```python
from build123d import *

# Parameters (mm, degrees)
CUT_EXTRUDE_1_DEPTH      = 168.620106193
SKETCH_3_R               = 9
CUT_EXTRUDE_2_DEPTH      = 163.450761771
PATTERN_CIRCULAR_1_COUNT = 6


with BuildPart() as part:
    # Эскиз1 → Повернуть1 (revolve)
    with BuildSketch(Plane.XY, mode=Mode.PRIVATE) as revolve_1_sk:
        Polygon((-90.5, 0), (-117.5, 0), (-117.5, -22), (-86.5, -22), (-86.5, -10), (-90.5, -10), align=None)
    revolve(revolve_1_sk.sketch.rotate(Axis((0, 22.934814099, 0), (0, -1, 0)), 270), axis=Axis((0, 22.934814099, 0), (0, -1, 0)))

    # Эскиз2 → Вырез-Вытянуть1 (cut, through all)
    with BuildSketch(Plane(origin=(0, 0, 0), x_dir=(1, 0, 0), z_dir=(0, 1, 0))):
        with BuildLine():
            Line((-110, 41.306779105), (-110, -41.306779105))
            ThreePointArc((-110, -41.306779105), (-117.5, 0), (-110, 41.306779105))
        make_face()
        with BuildLine():
            Line((110, 41.306779105), (110, -41.306779105))
            ThreePointArc((110, -41.306779105), (117.5, 0), (110, 41.306779105))
        make_face()
    extrude(amount=-CUT_EXTRUDE_1_DEPTH, mode=Mode.SUBTRACT)

    # Эскиз3 → Вырез-Вытянуть2 (cut, through all)
    with BuildSketch(Plane(origin=(0, 0, 0), x_dir=(1, 0, 0), z_dir=(0, 1, 0))):
        with Locations(Location((0, 102.5, 0), (0, 0, 270))):
            Circle(SKETCH_3_R)
    cut_extrude_2 = extrude(amount=-CUT_EXTRUDE_2_DEPTH, mode=Mode.SUBTRACT)

    # Круговой массив1: Вырез-Вытянуть2 ×6 about axis
    pattern_circular_1_axis = Axis((0, 0, 0), (0, 1, 0))
    for i in range(1, PATTERN_CIRCULAR_1_COUNT):
        add(cut_extrude_2.rotate(pattern_circular_1_axis, i * 360 / PATTERN_CIRCULAR_1_COUNT), mode=Mode.SUBTRACT)


solid = part.part
```
The listing builds one solid part. Answer for the finished solid, in the listing's coordinates (mm). A direction names the side the tool comes from. Give positions to 0.01 mm unless a question says otherwise; leave off trailing zeros. Write each loop counter-clockwise with the first axis right and the second up, starting at its lowest first coordinate (ties: lowest second). Pieces come first, ordered by that corner, then holes. Notation, with made-up numbers: M 59,11 L 109,11 A34 cw 109,41 Z; hole C -38.5,65.5 d7. An arc over 180 degrees is marked long. Write each question's results on one line, items separated by ' | '.
Q1. Flat-ended cylindrical pins translate along their axes: P1, Ø12, axis at x = 71, y = -19, coming from the -Z side; P2, Ø6, axis at y = -11, z = -78, coming from the -X side; P3, Ø5, axis at x = 36.5, y = -12.5, coming from the +Z side. Find the tip coordinate at first contact, or state that the pin passes through.
Output values:
P1: z = -97.88 | P2: x = -90.45 | P3: z = 112.47
Q2. Consider L1, parallel to X at y = -19.75, z = 57.5; L2, parallel to X at y = -11.25, z = -51.25; L3, parallel to X at y = -14.75, z = 0. Determine where each line is inside the solid, lowest interval first. Write a range as from..to.
Output values:
L1: -102.47..-95.24, -82.29..-64.62, 64.62..82.29, 95.24..102.47 | L2: -105.73..-97.77, -79.77..-69.68, 69.68..79.77, 97.77..105.73 | L3: -110..-86.5, 86.5..110
Q3. Section B-B, the plane x = -32.5 is taken. Write down the section's boundary in (y, z).
Output values:
outline: M -22,-112.92 L 0,-112.92 L 0,-84.46 L -10,-84.46 L -10,-80.16 L -22,-80.16 Z; M -22,80.16 L -10,80.16 L -10,84.46 L 0,84.46 L 0,112.92 L -22,112.92 Z
Q4. Section D-D, the plane y = -17 is taken. Write down the section's boundary in (x, z), then the cut area to 3 significant figures.
Output values:
outline: M -110,-41.31 A117.5 ccw 110,-41.31 L 110,41.31 A117.5 ccw -110,41.31 Z; hole C -88.77,-51.25 d18; hole C -88.77,51.25 d18; hole C 0,0 d173; hole C 0,-102.5 d18; hole C 0,102.5 d18; hole C 88.77,-51.25 d18; hole C 88.77,51.25 d18 | area: 17,500 mm2
Q5. Section A-A, the plane z = 0 is taken. Write down the section's boundary in (x, y), then the cut area to 3 significant figures.
Output values:
outline: M -110,-22 L -86.5,-22 L -86.5,-10 L -90.5,-10 L -90.5,0 L -110,0 Z; M 86.5,-22 L 110,-22 L 110,0 L 90.5,0 L 90.5,-10 L 86.5,-10 Z | area: 954 mm2
Q6. Section C-C, the plane z = 51.25 is taken. Write down the section's boundary in (x, y).
Output values:
outline: M -105.73,-22 L -97.77,-22 L -97.77,0 L -105.73,0 Z; M -79.77,-22 L -69.68,-22 L -69.68,-10 L -74.59,-10 L -74.59,0 L -79.77,0 Z; M 69.68,-22 L 79.77,-22 L 79.77,0 L 74.59,0 L 74.59,-10 L 69.68,-10 Z; M 97.77,-22 L 105.73,-22 L 105.73,0 L 97.77,0 Z
Q7. For a pull along X with two mould halves and no side action, classify faces 1 (the cylindrical face through (-82.68, -10.85, 44.62)), 2 (the flat face through (-90, 0, 18)), 3 (the cylindrical face through (1.993, -11.154, 117.483)) as released by +X, released by -X, zero draft, split by the parting line, or undercut.
Output values:
face 1: undercut | face 2: zero draft | face 3: split by the parting line
Q8. A tool of negligible diameter and unlimited length cuts with its end or side. For faces 4 (the cylindrical face through (88.37, -10.85, -42.26)), 5 (the cylindrical face through (-27.18, -4.93, 86.32)), from which of +Z, -Z, +X, -X, +Y, -Y can it reach the whole face along a straight path? Write none if from no direction.
Output values:
face 4: +Y, -Y | face 5: +Y
